For this review, take the finished solid that the model builds, in its own axes (mm). Face numbers are marked on the shaded views. A direction names the side the tool comes from. Round coordinates to 2 decimals unless told otherwise and drop trailing zeros. Loops run counter-clockwise (first coordinate to the right, second up) from the corner with the lowest first, then second, coordinate; pieces in that order, holes last.
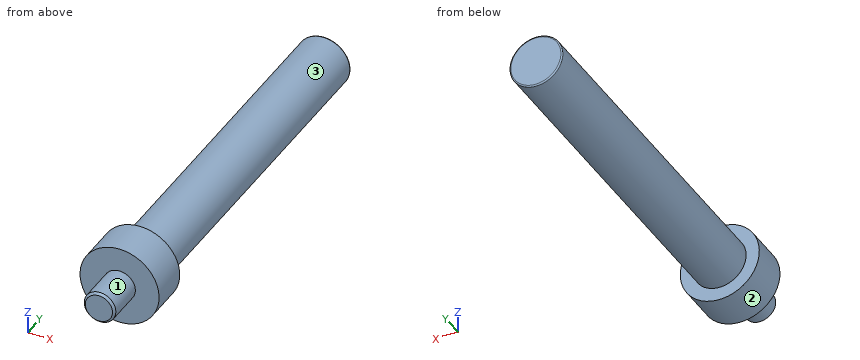
```python
from build123d import *

# Parameters (mm, degrees)
SKETCH1_R           = 15
BOSS_EXTRUDE1_DEPTH = 15
SKETCH2_R           = 10
BOSS_EXTRUDE2_DEPTH = 133.5
SKETCH4_R           = 7.5
BOSS_EXTRUDE3_DEPTH = 15
FILLET1_R           = 0.5


# Read off the part's stored shape, not the designer's step: M12x1.5 Machine Threads Stud1
with BuildPart() as part:
    # Sketch1 → Boss-Extrude1 (new body)
    with BuildSketch(Plane(origin=(0, 0, 0), x_dir=(1, 0, 0), z_dir=(0, 1, 0))):
        with Locations(Location((0, 0, 0), (0, 0, 270))):
            Circle(SKETCH1_R)
    extrude(amount=BOSS_EXTRUDE1_DEPTH)

    # Sketch2 → Boss-Extrude2 (add)
    with BuildSketch(Plane(origin=(0, 15, 0), x_dir=(1, 0, 0), z_dir=(0, 1, 0))):
        with Locations(Location((0, 0, 0), (0, 0, 270))):
            Circle(SKETCH2_R)
    extrude(amount=BOSS_EXTRUDE2_DEPTH)

    # Sketch4 → Boss-Extrude3 (add)
    with BuildSketch(Plane.XZ):
        with Locations(Location((0, 0, 0), (0, 0, 270))):
            Circle(SKETCH4_R)
    extrude(amount=BOSS_EXTRUDE3_DEPTH)

    # M12x1.5 Machine Threads Stud1 outline → M12x1.5 Machine Threads Stud1 (revolve, cut)
    with BuildSketch(Plane.XY):
        Polygon((7.5, 0), (6, 0), (6, -14.172), (5.172, -15), (7.5, -15), align=None)
    revolve(axis=Axis((0, 0, 0), (0, 1, 0)), mode=Mode.SUBTRACT)

    # Fillet1
    fillet1_edges = [part.edges().sort_by_distance(p)[0] for p in [
        (0, 148.5, -10),
    ]]
    fillet(fillet1_edges, radius=FILLET1_R)


solid = part.part
```
(1) Insertion check: pin 1 Ø10 at (x, y) = (-2.5, 129) entering from -Z; pin 2 Ø10 at (y, z) = (72.5, -2) entering from +X; pin 3 Ø3 at (y, z) = (100, 1) entering from -X. Each pin has a flat end and moves straight along its axis. Give the tip position at first contact, or say it passes through.
(2) For L1, parallel to Y at x = -13, z = -5.5; L2, parallel to Z at x = -0.5, y = 21; L3, parallel to Y at x = 8.25, z = 0, list the stretches that pass through material, from the lowest coordinate up.
(3) Add section B-B (z = 0). Give the boundary of the cut face in (x, y), plus the area to 3 significant figures.
(4) For the marked faces 1, 2 and 3, list the 3-axis set-ups (+Z, -Z, +X, -X, +Y, -Y) from which the entire face can be reached by the end or side of a thin tool; tool diameter is ignored.
(5) Add section D-D (x = 12). Give the boundary of the cut face in (y, z), plus the area to 3 significant figures.
(6) Add section A-A (x = 0). Give the boundary of the cut face in (y, z).
(7) Add section C-C (y = 13). Give the boundary of the cut face in (x, z).
Outcome:
1. pin 1: stops at z = -10
1. pin 2: stops at x = 10
1. pin 3: stops at x = -10
2. L1: y = 0 to 15
2. L2: z = -9.99 to 9.99
2. L3: y = 0 to 148.5
3. outline: (-15, 0) - (-6, 0) - (-6, -14.17) - (-5.17, -15) - (5.17, -15) - (6, -14.17) - (6, 0) - (15, 0) - (15, 15) - (10, 15) - (10, 148) arc R0.5 ccw to (9.5, 148.5) - (-9.5, 148.5) arc R0.5 ccw to (-10, 148) - (-10, 15) - (-15, 15) - close
3. area: 3,300 mm2
4. face 1: -Y
4. face 2: +Y, -Y
4. face 3: +Y
5. outline: (0, -9) - (15, -9) - (15, 9) - (0, 9) - close
5. area: 270 mm2
6. outline: (-15, -5.17) - (-14.17, -6) - (0, -6) - (0, -15) - (15, -15) - (15, -10) - (148, -10) arc R0.5 ccw to (148.5, -9.5) - (148.5, 9.5) arc R0.5 ccw to (148, 10) - (15, 10) - (15, 15) - (0, 15) - (0, 6) - (-14.17, 6) - (-15, 5.17) - close
7. outline: circle Ø30 at (0, 0)
